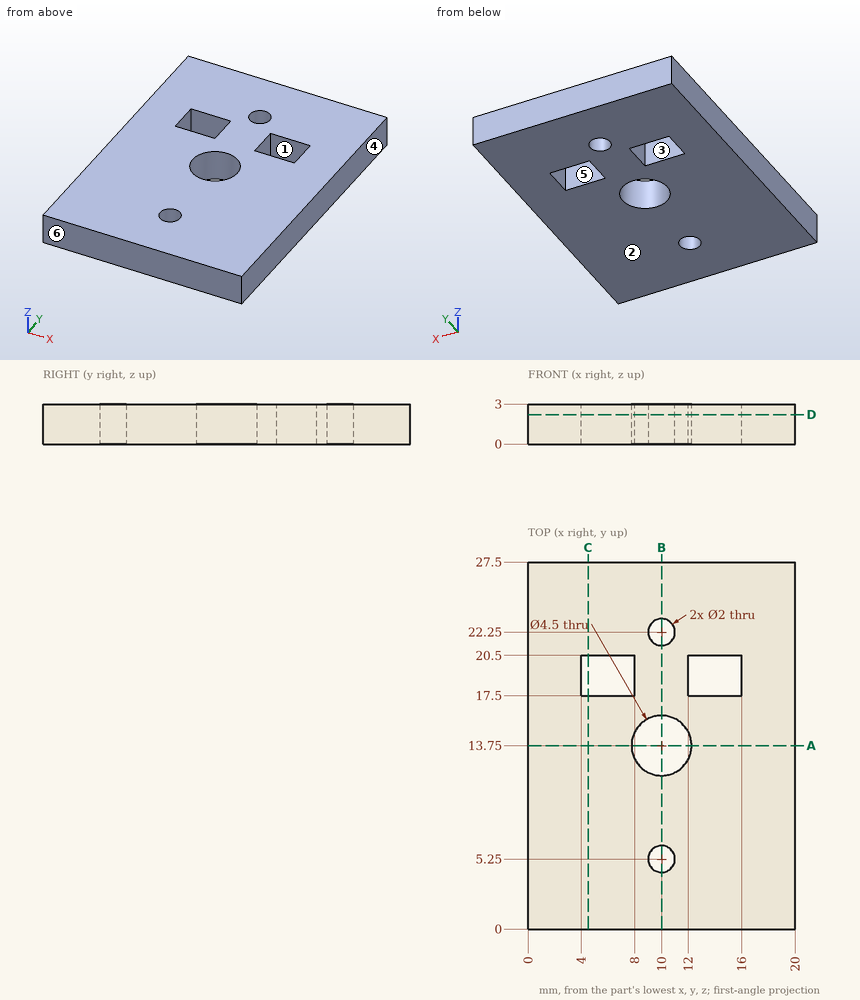
Geometry check sheet. Reference: drawing and pictorial views, mm from the part's lowest x, y, z. A direction names the side the tool comes from. Give positions to 0.01 mm unless a question says otherwise; leave off trailing zeros. Order: outer loops, then holes, each group sorted by start corner. A loop starts at its lowest first (then second) coordinate and runs counter-clockwise, first axis right, second up.
1. Thickness scan on L1, parallel to X at y = 20, z = 2.5; L2, parallel to Y at x = 10, z = 2.3; L3, parallel to Y at x = 15, z = 1.3. Record the ranges inside material, lowest first.
2. Release check for a two-part mould opening along X. For the marked faces 1, 2, 3 and 4 record: pulls with the +X half, pulls with the -X half, needs draft (parallel to the pull), parting line crosses it, or undercut.
3. Access from +Z, -Z, +X, -X, +Y, -Y to the whole of each face (thin tool, end or side, straight path). Record for the marked faces 5 and 6.
4. Gauge pin test, flat end, axial feed: pin 1 Ø1.2 at (x, y) = (10, 22.25) entering from -Z. Record the tip position at first contact, or that the pin passes through.
5. Section check B-B, the plane x = 10. Enter the section's corners in (y, z), and give its area (3 significant figures).
6. Section check D-D, the plane z = 2.2. Enter the section's corners in (x, y), and give its area (3 significant figures).
7. Section check C-C, the plane x = 4.5. Enter the section's corners in (y, z), and give its area (3 significant figures).
8. Section check A-A, the plane y = 13.75. Enter the section's corners in (x, z), and give its area (3 significant figures).
Values follow:
1. L1: x = 0 to 4, 8 to 12, 16 to 20
1. L2: y = 0 to 4.25, 6.25 to 11.5, 16 to 21.25, 23.25 to 27.5
1. L3: y = 0 to 17.5, 20.5 to 27.5
2. face 1: undercut
2. face 2: needs draft
2. face 3: undercut
2. face 4: pulls with the +X half
3. face 5: +Z, -Z
3. face 6: +Z, -Z, +X, -X, -Y
4. pin 1: passes through
5. outline: (0, 0) - (4.25, 0) - (4.25, 3) - (0, 3) - close; (6.25, 0) - (11.5, 0) - (11.5, 3) - (6.25, 3) - close; (16, 0) - (21.25, 0) - (21.25, 3) - (16, 3) - close; (23.25, 0) - (27.5, 0) - (27.5, 3) - (23.25, 3) - close
5. area: 57.0 mm2
6. outline: (0, 0) - (20, 0) - (20, 27.5) - (0, 27.5) - close; hole (4, 17.5) - (8, 17.5) - (8, 20.5) - (4, 20.5) - close; hole circle Ø4.5 at (10, 13.75); hole circle Ø2 at (10, 5.25); hole circle Ø2 at (10, 22.25); hole (12, 17.5) - (16, 17.5) - (16, 20.5) - (12, 20.5) - close
6. area: 504 mm2
7. outline: (0, 0) - (17.5, 0) - (17.5, 3) - (0, 3) - close; (20.5, 0) - (27.5, 0) - (27.5, 3) - (20.5, 3) - close
7. area: 73.5 mm2
8. outline: (0, 0) - (7.75, 0) - (7.75, 3) - (0, 3) - close; (12.25, 0) - (20, 0) - (20, 3) - (12.25, 3) - close
8. area: 46.5 mm2
